Verification items for the finished model (mm, model axes). Face numbers are marked on the shaded views. A direction names the side the tool comes from. Coordinates: 2 decimals unless noted, no trailing zeros. Order: outer loops, then holes, each group sorted by start corner. A loop starts at its lowest first (then second) coordinate and runs counter-clockwise, first axis right, second up. Notation, with made-up numbers: M 58,14.25 L 105,14.25 A30 ccw 105,40.25 Z; hole C 82,67 d3. An arc over 180 degrees is marked long. Return JSON: item names as keys, results as strings.
Autodesk Inventor part; units mm, degrees
ref_plane "YZ Plane" through (0, 0, 0) normal (1, 0, 0) x (0, 1, 0)
ref_plane "XZ Plane" through (0, 0, 0) normal (0, 1, 0) x (-1, 0, 0)
ref_plane "XY Plane" through (0, 0, 0) normal (0, 0, 1) x (1, 0, 0)
sketch "Sketch1" plane through (0, 0, 0) normal (0, 0, 1) x (1, 0, 0)
  line L0 (0, 0) -> (43, 0)
  line L1 (43, 0) -> (43, 21.5)
  line L2 (43, 21.5) -> (0, 21.5)
  line L3 (0, 21.5) -> (0, 0)
  dimension "d0" = 43
  dimension "d1" = 21.5
  dimension "d2" = 43
extrude "Extrusion1" add sketch "Sketch1" along normal blind 1.1
sketch "Sketch2" plane through (0, 0, 1.1) normal (0, 0, 1) x (1, 0, 0)
  line L0 (43, 21.5) -> (0, 21.5)
  line L1 (0, 21.5) -> (6.5, 21.5)
  line L2 (6.5, 21.5) -> (6.5, 19)
  circle A0 centre (6.5, 19) radius 1.5
  line L3 (0, 0) -> (43, 0)
  line L4 (43, 0) -> (36.5, 0)
  line L5 (36.5, 0) -> (36.5, 2.5)
  circle A1 centre (36.5, 2.5) radius 1.5
  dimension "d5" = 6.5
  dimension "d6" = 2.5
  dimension "d7" = 3
  dimension "d8" = 6.5
  dimension "d9" = 2.5
  dimension "d10" = 3
extrude "Extrusion2" cut sketch "Sketch2" against normal blind 1.1
sketch "Sketch3" plane through (0, 0, 1.1) normal (0, 0, 1) x (1, 0, 0)
  circle A0 centre (4.6207, 9.3261) radius 3.5
  circle A1 centre (38.2496, 10.1463) radius 3.5
  point P0 (0, 0)
  dimension "d13" = 7
  dimension "d14" = 7
extrude "Extrusion3" add sketch "Sketch3" along normal blind 10
sketch "Sketch4" plane through (0, 0, 1.1) normal (0, 0, 1) x (1, 0, 0)
  line L0 (31.8145, 20.2348) -> (31.8145, 17.4683)
  line L1 (31.8145, 17.4683) -> (22.3294, 17.4683)
  line L2 (22.3294, 17.4683) -> (22.3294, 20.2348)
  line L3 (22.3294, 20.2348) -> (31.8145, 20.2348)
  point P0 (0, 0)
extrude "Extrusion4" add sketch "Sketch4" along normal blind 11
sketch "Sketch5" plane through (0, 0, 1.1) normal (0, 0, 1) x (1, 0, 0)
  line L0 (31.4983, 11.4611) -> (31.4983, 1.7389)
  line L1 (31.4983, 1.7389) -> (20.1953, 1.7389)
  line L2 (20.1953, 1.7389) -> (20.1953, 11.4611)
  line L3 (20.1953, 11.4611) -> (31.4983, 11.4611)
  point P0 (0, 0)
extrude "Extrusion5" add sketch "Sketch5" along normal blind 8
sketch "Sketch6" plane through (0, 0, 1.1) normal (0, 0, 1) x (1, 0, 0)
  line L0 (9.0495, 18.4071) -> (19.8493, 18.4071)
  line L1 (19.8493, 18.4071) -> (19.8493, 12.5444)
  line L2 (19.8493, 12.5444) -> (9.0495, 12.5444)
  line L3 (9.0495, 12.5444) -> (9.0495, 18.4071)
  point P0 (0, 0)
extrude "Extrusion6" add sketch "Sketch6" along normal blind 3
properties part number "VoltageRegulator"
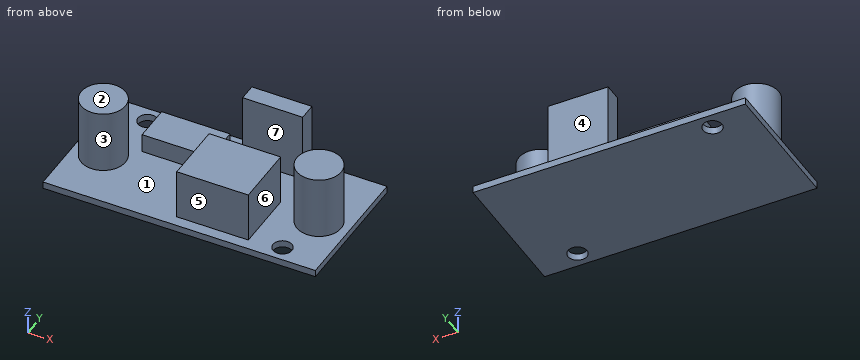
Q1. Cross-section at C-C, the plane x = 7.5. Record the boundary of the cut face in (y, z), and give its area (3 significant figures).
Values:
{"outline": "M 0,0 L 17.88,0 L 17.88,1.1 L 11.32,1.1 L 11.32,11.1 L 7.34,11.1 L 7.34,1.1 L 0,1.1 Z; M 20.12,0 L 21.5,0 L 21.5,1.1 L 20.12,1.1 Z", "area": "61.0 mm^2"}
Q2. Material ranges on line 1 along X through (y, z) = (19, 0.65); line 2 along Y through (x, z) = (29.5, 1.5); line 3 along Y through (x, z) = (6.5, 0.55), recorded low to high.
Values:
{"line 1": "0 to 5, 8 to 43", "line 2": "1.74 to 11.46, 17.47 to 20.23", "line 3": "0 to 17.5, 20.5 to 21.5"}
Q3. Cross-section at A-A, the plane y = 2.5. Record the boundary of the cut face in (x, z), and give its area (3 significant figures).
Values:
{"outline": "M 0,0 L 35,0 L 35,1.1 L 31.5,1.1 L 31.5,9.1 L 20.2,9.1 L 20.2,1.1 L 0,1.1 Z; M 38,0 L 43,0 L 43,1.1 L 38,1.1 Z", "area": "134 mm^2"}
Q4. Tool access check on the marked faces 3, 4, 5, 6 and 7. Record the directions out of +Z, -Z, +X, -X, +Y, -Y that give a thin tool (end or side, any length) a straight path to the whole face; none if there is none.
Values:
{"face 3": "+Z", "face 4": "+Z, +X, -X, +Y", "face 5": "+Z, +X, -X, -Y", "face 6": "+Z, -Y", "face 7": "+Z, +X"}
Q5. Cross-section at B-B, the plane z = 8. Record the boundary of the cut face in (x, y), and give its area (3 significant figures).
Values:
{"outline": "C 4.62,9.33 d7; M 20.2,1.74 L 31.5,1.74 L 31.5,11.46 L 20.2,11.46 Z; M 22.33,17.47 L 31.81,17.47 L 31.81,20.23 L 22.33,20.23 Z; C 38.25,10.15 d7", "area": "213 mm^2"}
Q6. Go/stop test with flat-tipped pins: pin 1 (2 mm diameter, centred on x = 39, y = 9.5, fed in from +Z); pin 2 (2 mm diameter, centred on x = 29, y = 4, fed in from +Z); pin 3 (6.5 mm diameter, centred on y = 5, z = 6.5, fed in from -X); pin 4 (3 mm diameter, centred on x = 18.5, z = 7, fed in from -Y). Record where each tip stops, or that it passes through.
Values:
{"pin 1": "z = 11.1", "pin 2": "z = 9.1", "pin 3": "x = 1.29", "pin 4": "through"}
Q7. Cross-section at D-D, the plane x = 14.5. Record the boundary of the cut face in (y, z), and give its area (3 significant figures).
Values:
{"outline": "M 0,0 L 21.5,0 L 21.5,1.1 L 18.41,1.1 L 18.41,4.1 L 12.54,4.1 L 12.54,1.1 L 0,1.1 Z", "area": "41.2 mm^2"}
Q8. Draft check along X on the marked faces 1 and 2. Enter one of: pulls with the +X half, pulls with the -X half, needs draft (parallel to the pull), parting line crosses it, or undercut.
Values:
{"face 1": "undercut", "face 2": "needs draft"}
